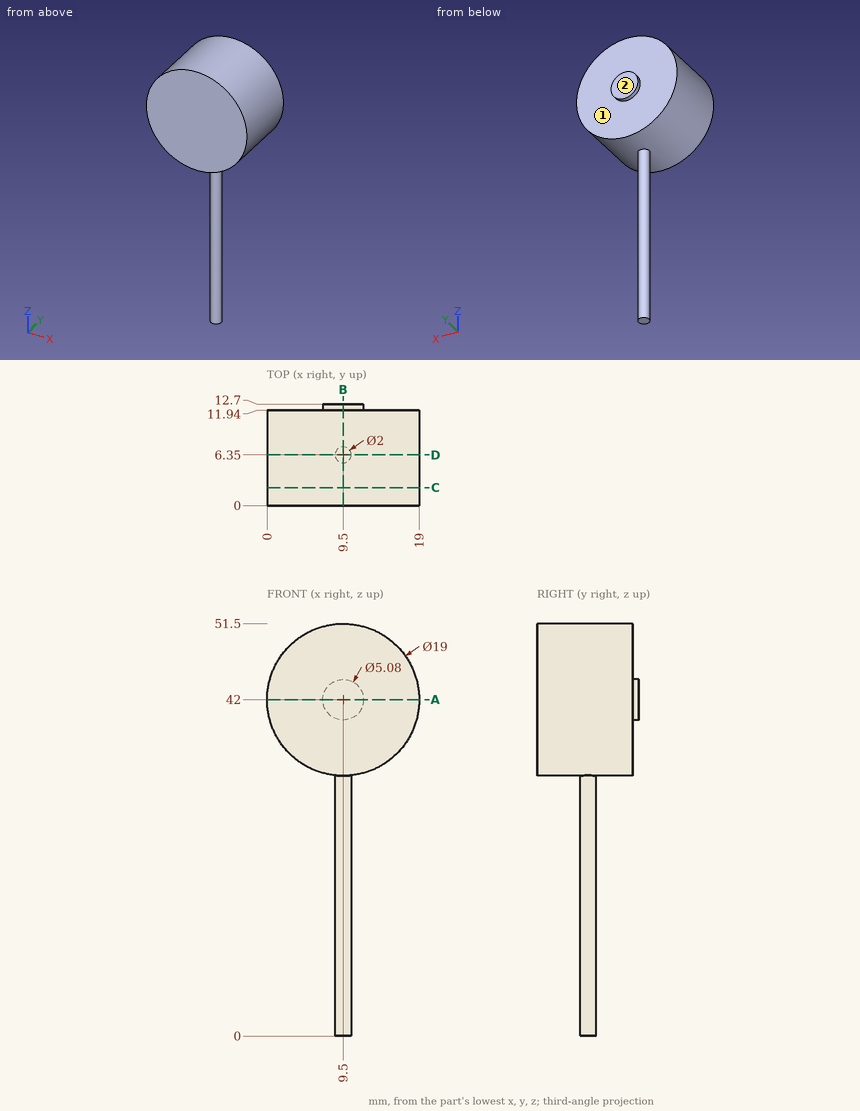
Here's the drawing with two shaded views (mm, measured from the low corner). I have some questions. A direction names the side the tool comes from. Coordinates: 2 decimals unless noted, no trailing zeros. Write each loop counter-clockwise with the first axis right and the second up, starting at its lowest first coordinate (ties: lowest second). Pieces come first, ordered by that corner, then holes.
Item 1: Will these pins go through, and if not, where does the flat tip stop? pin 1 (3 mm diameter, centred on x = 6.5, y = 2.5, fed in from -Z); pin 2 (6 mm diameter, centred on x = 15, y = 10, fed in from +Z); pin 3 (6 mm diameter, centred on y = 4, z = 46, fed in from -X).
Item 2: I want a section at A-A on z = 42. Write out the boundary of the cut face in (x, y), and give its area (3 significant figures).
Item 3: On a 3-axis mill with a long thin cutter (end or side, diameter ignored), from which of +Z, -Z, +X, -X, +Y, -Y can I reach the whole of each face in a straight line? I mean the marked faces 1 and 2. Say none if no direction works.
Item 4: I want a section at C-C on y = 2.25. Write out the boundary of the cut face in (x, z).
Item 5: I want a section at D-D on y = 6.35. Write out the boundary of the cut face in (x, z).
Item 6: If I drill on line 1 (Y direction, x = 14.25, z = 49); line 2 (Z direction, x = 9.75, y = 10); line 3 (Y direction, x = 10.25, z = 9), over which ranges is the centre line in solid material (lowest first)?
Item 7: I want a section at B-B on x = 9.5. Write out the boundary of the cut face in (y, z), and give its area (3 significant figures).
Findings below:
1. pin 1: stops at z = 32.62
1. pin 2: stops at z = 51.17
1. pin 3: stops at x = 0.05
2. outline: (0, 0) - (19, 0) - (19, 11.94) - (12.04, 11.94) - (12.04, 12.7) - (6.96, 12.7) - (6.96, 11.94) - (0, 11.94) - close
2. area: 231 mm2
3. face 1: +Y
3. face 2: +Z, -Z, +X, -X, +Y
4. outline: circle Ø19 at (9.5, 42)
5. outline: (8.5, 0) - (10.5, 0) - (10.5, 32.55) arc R9.5 ccw (long way) to (8.5, 32.55) - close
6. line 1: y = 0 to 11.94
6. line 2: z = 32.5 to 51.5
6. line 3: y = 5.69 to 7.01
7. outline: (0, 32.5) - (5.35, 32.5) - (5.35, 0) - (7.35, 0) - (7.35, 32.5) - (11.94, 32.5) - (11.94, 39.46) - (12.7, 39.46) - (12.7, 44.54) - (11.94, 44.54) - (11.94, 51.5) - (0, 51.5) - close
7. area: 296 mm2
